```python
from build123d import *

# Parameters (mm, degrees)
SKETCH1_W               = 83
SKETCH1_H               = 65
BASE_FLANGE1_DEPTH      = 2
SKETCH6_R               = 9.05
CUT_EXTRUDE1_DEPTH      = 12
M3_CLEARANCE_HOLE1_D    = 3.4
LPATTERN1_COUNT         = 2
LPATTERN1_PITCH         = 33
FILLET1_R               = 5
FLAT_PATTERN1_START     = -2
FLAT_PATTERN1_OUTLINE_R = 2.75
FLAT_PATTERN1_DEPTH     = 2


# Read off the part's stored shape, not the designer's step: Flat-Pattern1
# Sheet-metal steps are written as plain solids
with BuildPart() as part:
    # Sketch1 → Base-Flange1 (new body)
    with BuildSketch(Plane.XY):
        Rectangle(SKETCH1_W, SKETCH1_H)
    extrude(amount=-BASE_FLANGE1_DEPTH)

    # Sketch6 → Cut-Extrude1 (cut)
    with BuildSketch(Plane.XY):
        with Locations((16.541079456, 11.5)):
            Circle(SKETCH6_R)
        with Locations((-16.458920544, 11.5)):
            Circle(SKETCH6_R)
    extrude(amount=-CUT_EXTRUDE1_DEPTH, mode=Mode.SUBTRACT)

    # M3 Clearance Hole1 (through all)
    with Locations(Plane.XY):
        with Locations((16.50520677, 22.499941507), (27.541020963, 11.535872686), (5.541137949, 11.464127314), (16.576952141, 0.500058493)):
            m3_clearance_hole1 = Hole(M3_CLEARANCE_HOLE1_D / 2)

    # LPattern1: M3 Clearance Hole1 ×2
    with Locations(*[(-i * LPATTERN1_PITCH, 0, 0) for i in range(1, LPATTERN1_COUNT)]):
        add(m3_clearance_hole1, mode=Mode.SUBTRACT)

    # Fillet1
    fillet1_edges = [part.edges().sort_by_distance(p)[0] for p in [
        (41.5, -32.5, -1),
        (-41.5, -32.5, -1),
        (-41.5, 32.5, -1),
        (41.5, 32.5, -1),
    ]]
    fillet(fillet1_edges, radius=FILLET1_R)

    # Flat-Pattern1 outline → Flat-Pattern1 (cut)
    with BuildSketch(Plane.XY.offset(FLAT_PATTERN1_START)):
        with Locations((-21.496938457, -23.5)):
            Circle(FLAT_PATTERN1_OUTLINE_R)
        with Locations((21.5, -23.5)):
            Circle(FLAT_PATTERN1_OUTLINE_R)
    extrude(amount=FLAT_PATTERN1_DEPTH, mode=Mode.SUBTRACT)


solid = part.part
```
The listing builds one solid part. Answer for the finished solid, in the listing's coordinates (mm). Round coordinates to 2 decimals unless told otherwise and drop trailing zeros. Write each loop counter-clockwise with the first axis right and the second up, starting at its lowest first coordinate (ties: lowest second). Pieces come first, ordered by that corner, then holes. Notation, with made-up numbers: (12, -6) -> (31, -6) arc R15 ccw to (31, 9) -> close; hole circle Ø4 at (65, 17). An arc over 180 degrees is marked (long way). Use CSV: the item, a comma, the result in double quotes. Start each with the question number.
(1) Section B-B on x = 5 is taken. Give the vertices of the cut face in (y, z), then the cut area to 3 significant figures.
(2) The mould has two halves that part along Y. Classify faces 1 (the face through (-40.07, 31, -1.01)), 2 (the face through (-15.146, 21.466, -1.014)), 3 (the face through (41.5, 0, -1)), 4 (the face through (-17.993, -0.151, -1.014)): released by +Y, released by -Y, zero draft, split by the parting line, or undercut.
(3) Section C-C on x = 21.5 is taken. Give the vertices of the cut face in (y, z).
(4) Section A-A on y = -23.5 is taken. Give the vertices of the cut face in (x, z).
(5) Section D-D on z = -1.7 is taken. Count the separate pieces of the cut face and the enclosed holes in it, then the cut area to 3 significant figures.
(6) Consider L1, parallel to Y at x = 18, z = -1.4; L2, parallel to X at y = 21.5, z = -0.5; L3, parallel to Y at x = 21.5, z = -0.95. Determine where each line is inside the solid, lowest interval first. Write a range as from..to.
A:
1,outline,"(-32.5, -2) -> (9.85, -2) -> (9.85, 0) -> (-32.5, 0) -> close; (13.08, -2) -> (32.5, -2) -> (32.5, 0) -> (13.08, 0) -> close"
1,area,"124 mm²"
2,face 1,"released by +Y"
2,face 2,"undercut"
2,face 3,"zero draft"
2,face 4,"undercut"
3,outline,"(-32.5, -2) -> (-26.25, -2) -> (-26.25, 0) -> (-32.5, 0) -> close; (-20.75, -2) -> (3.93, -2) -> (3.93, 0) -> (-20.75, 0) -> close; (19.07, -2) -> (32.5, -2) -> (32.5, 0) -> (19.07, 0) -> close"
4,outline,"(-41.5, -2) -> (-24.25, -2) -> (-24.25, 0) -> (-41.5, 0) -> close; (-18.75, -2) -> (18.75, -2) -> (18.75, 0) -> (-18.75, 0) -> close; (24.25, -2) -> (41.5, -2) -> (41.5, 0) -> (24.25, 0) -> close"
5,separate pieces,"1"
5,enclosed holes,"12"
5,area,"4,740 mm²"
6,L1,"y = -32.5..-0.43, 1.43..2.57, 20.43..21.69, 23.31..32.5"
6,L2,"x = -41.5..-17.87, -15.12..15.13, 17.88..41.5"
6,L3,"y = -32.5..-26.25, -20.75..3.93, 19.07..32.5"
